For this review, take the finished solid that the model builds, in its own axes (mm). A direction names the side the tool comes from. Give positions to 0.01 mm unless a question says otherwise; leave off trailing zeros. Order: outer loops, then holes, each group sorted by start corner. A loop starts at its lowest first (then second) coordinate and runs counter-clockwise, first axis right, second up. Notation, with made-up numbers: (64, -39) -> (75, -39) arc R16 ccw to (75, -23) -> close; hole circle Ø11 at (27.5, -16.5). An arc over 180 degrees is marked (long way). Return JSON: item names as keys, results as strings. Group by question number.
1) Add section B-B (z = 3). Give the boundary of the cut face in (x, y).
2) Add section A-A (x = 14). Give the boundary of the cut face in (y, z).
3) To check wall thickness, follow line 1 along Z through (x, y) = (22, 5); line 2 along Y through (x, z) = (13.25, 0.85); line 3 along X through (y, z) = (21.5, 5.05). State the ranges of each line that lie inside material, in increasing order.
4) The part is to be moulded in two halves that separate along Z. For faces 1 (the face through (6, 10, 3)), 2 (the face through (14, 13, 6)), 3 (the face through (0, 9, 3)), 4 (the face through (14, 13, 0)), say which applies: released by +Z, released by -Z, zero draft, split by the parting line, or undercut.
5) Add section D-D (y = 23). Give the boundary of the cut face in (x, z).
6) For faces 5 (the face through (23.22, 4.93, 2.73)), 6 (the face through (14, 32, 3)), list the 3-axis set-ups (+Z, -Z, +X, -X, +Y, -Y) from which the entire face can be reached by the end or side of a thin tool; tool diameter is ignored.
7) Add section C-C (y = 6). Give the boundary of the cut face in (x, z), then the cut area to 3 significant figures.
8) Insertion check: P1, Ø3, axis at x = 6, z = 3, coming from the +Y side; P2, Ø1.5, axis at x = 18, z = 5.5, coming from the +Y side; P3, Ø1.5, axis at x = 22, z = 3, coming from the -Y side. Each pin has a flat end and moves straight along its axis. Give the tip position at first contact, or say it passes through.
from build123d import *

# Parameters (mm, degrees)
ESQUISSE1_W             = 28
ESQUISSE1_H             = 32
BOSS_EXTRU_1_DEPTH      = 6
ESQUISSE2_R             = 1.25
ENL_V_MAT_EXTRU_1_DEPTH = 10
ESQUISSE3_R             = 5.5
ENL_V_MAT_EXTRU_2_DEPTH = 43.941821107
ESQUISSE4_R             = 1
ENL_V_MAT_EXTRU_4_DEPTH = 43.941821107
ENL_V_MAT_EXTRU_5_DEPTH = 43.941821107


with BuildPart() as part:
    # Esquisse1 → Boss.-Extru.1 (new body)
    with BuildSketch(Plane.XY):
        with Locations((14, 16)):
            Rectangle(ESQUISSE1_W, ESQUISSE1_H)
    extrude(amount=BOSS_EXTRU_1_DEPTH)

    # Esquisse2 → Enlèv. mat.-Extru.1 (cut)
    with BuildSketch(Plane.XZ):
        with Locations(Location((6, 3, 0), (0, 0, 270))):
            Circle(ESQUISSE2_R)
        with Locations(Location((22, 3, 0), (0, 0, 90))):
            Circle(ESQUISSE2_R)
    extrude(amount=-ENL_V_MAT_EXTRU_1_DEPTH, mode=Mode.SUBTRACT)

    # Esquisse3 → Enlèv. mat.-Extru.2 (cut, through all)
    with BuildSketch(Plane.XY.offset(6)):
        with Locations((14, 19)):
            Circle(ESQUISSE3_R)
    extrude(amount=-ENL_V_MAT_EXTRU_2_DEPTH, mode=Mode.SUBTRACT)

    # Esquisse4 → Enlèv. mat.-Extru.4 (cut, through all)
    with BuildSketch(Plane.XY.offset(6)):
        with Locations((14, 10)):
            Circle(ESQUISSE4_R)
        with Locations((5, 19)):
            Circle(ESQUISSE4_R)
        with Locations((14, 28)):
            Circle(ESQUISSE4_R)
        with Locations((23, 19)):
            Circle(ESQUISSE4_R)
    extrude(amount=-ENL_V_MAT_EXTRU_4_DEPTH, mode=Mode.SUBTRACT)

    # Esquisse5 → Enlèv. mat.-Extru.5 (cut, through all)
    with BuildSketch(Plane.XY.offset(6)):
        with BuildLine():
            Line((0, 19), (0, 33))
            Line((0, 33), (28, 33))
            Line((28, 33), (28, 19))
            ThreePointArc((28, 19), (14, 32), (0, 19))
        make_face()
    extrude(amount=-ENL_V_MAT_EXTRU_5_DEPTH, mode=Mode.SUBTRACT)


solid = part.part
Evaluation:
{
 "1": {"outline": "(0, 0) -> (4.75, 0) -> (4.75, 10) -> (7.25, 10) -> (7.25, 0) -> (20.75, 0) -> (20.75, 10) -> (23.25, 10) -> (23.25, 0) -> (28, 0) -> (28, 19) arc R14.04 ccw to (0, 19) -> close; hole circle Ø2 at (5, 19); hole circle Ø11 at (14, 19); hole circle Ø2 at (14, 10); hole circle Ø2 at (14, 28); hole circle Ø2 at (23, 19)"},
 "2": {"outline": "(0, 0) -> (9, 0) -> (9, 6) -> (0, 6) -> close; (11, 0) -> (13.5, 0) -> (13.5, 6) -> (11, 6) -> close; (24.5, 0) -> (27, 0) -> (27, 6) -> (24.5, 6) -> close; (29, 0) -> (32, 0) -> (32, 6) -> (29, 6) -> close"},
 "3": {"line 1": "0 to 1.75, 4.25 to 6", "line 2": "0 to 9.34, 10.66 to 13.55, 24.45 to 27.34, 28.66 to 31.98", "line 3": "0.41 to 9.1, 18.9 to 27.59"},
 "4": {"face 1": "undercut", "face 2": "released by +Z", "face 3": "zero draft", "face 4": "released by -Z"},
 "5": {"outline": "(0.9, 0) -> (10.23, 0) -> (10.23, 6) -> (0.9, 6) -> close; (17.77, 0) -> (27.1, 0) -> (27.1, 6) -> (17.77, 6) -> close"},
 "6": {"face 5": "-Y", "face 6": "+Z, -Z, +Y"},
 "7": {"outline": "(0, 0) -> (28, 0) -> (28, 6) -> (0, 6) -> close; hole circle Ø2.5 at (6, 3); hole circle Ø2.5 at (22, 3)", "area": "158 mm^2"},
 "8": {"P1": "y = 30.4", "P2": "y = 31.62", "P3": "y = 10"}
}
